```python
from build123d import *

# Parameters (mm, degrees)
SKETCH_1_R            = 4.5
EXTRUDE_1_DEPTH       = 2.5
SKETCH_2_W            = 10
SKETCH_2_H            = 10
EXTRUDE_2_DEPTH       = 1.5
SKETCH_3_W            = 1.5
SKETCH_3_H            = 10
EXTRUDE_3_DEPTH       = 2
HOLE_WIZARD_3_0_3_1_D = 3


with BuildPart() as part:
    # 草圖1 → 填料-伸長1 (new body)
    with BuildSketch(Plane.XY):
        Circle(SKETCH_1_R)
    extrude(amount=EXTRUDE_1_DEPTH)

    # 草圖2 → 填料-伸長2 (add)
    with BuildSketch(Plane.XY.offset(2.5)):
        Rectangle(SKETCH_2_W, SKETCH_2_H)
    extrude(amount=EXTRUDE_2_DEPTH)

    # 草圖3 → 填料-伸長3 (add)
    with BuildSketch(Plane.XY.offset(4)):
        with Locations((-4.25, 0)):
            Rectangle(SKETCH_3_W, SKETCH_3_H)
    extrude_3 = extrude(amount=EXTRUDE_3_DEPTH)

    # 鏡射1: 填料-伸長3 across plane
    add(extrude_3.mirror(Plane(origin=(0, 0, 0), x_dir=(0, 0, 1), z_dir=(1, 0, 0))))

    # Ø3.0 (3) 直徑孔1 (through all)
    with Locations(Plane.XY.offset(4)):
        with Locations((0, 0)):
            Hole(HOLE_WIZARD_3_0_3_1_D / 2)


solid = part.part
```
Verification items for the finished model (mm, model axes). A direction names the side the tool comes from. Give positions to 0.01 mm unless a question says otherwise; leave off trailing zeros. Order: outer loops, then holes, each group sorted by start corner. A loop starts at its lowest first (then second) coordinate and runs counter-clockwise, first axis right, second up. Notation, with made-up numbers: (14, 27.25) -> (23, 27.25) arc R30 ccw to (23, 57.25) -> close; hole circle Ø10 at (12, 31.25). An arc over 180 degrees is marked (long way). Use a Markdown table: item, result.
1) Section check A-A, the plane y = 0. Record the boundary of the cut face in (x, z).
Results:
| item | result |
|---|---|
| outline | (-5, 2.5) -> (-4.5, 2.5) -> (-4.5, 0) -> (-1.5, 0) -> (-1.5, 4) -> (-3.5, 4) -> (-3.5, 6) -> (-5, 6) -> close; (1.5, 0) -> (4.5, 0) -> (4.5, 2.5) -> (5, 2.5) -> (5, 6) -> (3.5, 6) -> (3.5, 4) -> (1.5, 4) -> close |
2) Tool access check on faces 1 (the flat face through (3.5, 0, 5)), 2 (the flat face through (-1.2, 4.5, 2.5)), 3 (the flat face through (-4, 0, 6)). Record the directions out of +Z, -Z, +X, -X, +Y, -Y that give a thin tool (end or side, any length) a straight path to the whole face; none if there is none.
Results:
| item | result |
|---|---|
| face 1 | +Z, +Y, -Y |
| face 2 | -Z |
| face 3 | +Z, +X, -X, +Y, -Y |
3) Material ranges on probe 1 along X at (y, z) = (-3.25, 4.05); probe 2 along Y at (x, z) = (0, 2.8); probe 3 along Y at (x, z) = (0, 2.05), recorded low to high.
Results:
| item | result |
|---|---|
| probe 1 | -5 to -3.5, 3.5 to 5 |
| probe 2 | -5 to -1.5, 1.5 to 5 |
| probe 3 | -4.5 to -1.5, 1.5 to 4.5 |
4) Depth check by flat-ended pin: pin 1 Ø1 at (x, z) = (-0.5, 1.5) entering from -Y; pin 2 Ø1.8 at (x, y) = (0, 0) entering from -Z. Enter the tip coordinate at first touch or a pass-through.
Results:
| item | result |
|---|---|
| pin 1 | y = -4.5 |
| pin 2 | through |
5) Section check D-D, the plane x = -2.25. Record the boundary of the cut face in (y, z), then the cut area to 3 significant figures.
Results:
| item | result |
|---|---|
| outline | (-5, 2.5) -> (-3.9, 2.5) -> (-3.9, 0) -> (3.9, 0) -> (3.9, 2.5) -> (5, 2.5) -> (5, 4) -> (-5, 4) -> close |
| area | 34.5 mm² |
6) Mould release check, pull along X, two halves, no side actions. Record for faces 4 (the flat face through (4, 0, 6)), 5 (the cylindrical face through (-0.59, 4.46, 1.23)), 6 (the flat face through (-2, 0, 4)), 7 (the flat face through (-3.5, 0, 5)): pulls with the +X half, pulls with the -X half, needs draft (parallel to the pull), parting line crosses it, or undercut.
Results:
| item | result |
|---|---|
| face 4 | needs draft |
| face 5 | parting line crosses it |
| face 6 | undercut |
| face 7 | undercut |
7) Section check C-C, the plane z = 2.8. Record the boundary of the cut face in (x, y), then the cut area to 3 significant figures.
Results:
| item | result |
|---|---|
| outline | (-5, -5) -> (5, -5) -> (5, 5) -> (-5, 5) -> close; hole circle Ø3 at (0, 0) |
| area | 92.9 mm² |
8) Section check B-B, the plane x = 0. Record the boundary of the cut face in (y, z).
Results:
| item | result |
|---|---|
| outline | (-5, 2.5) -> (-4.5, 2.5) -> (-4.5, 0) -> (-1.5, 0) -> (-1.5, 4) -> (-5, 4) -> close; (1.5, 0) -> (4.5, 0) -> (4.5, 2.5) -> (5, 2.5) -> (5, 4) -> (1.5, 4) -> close |
